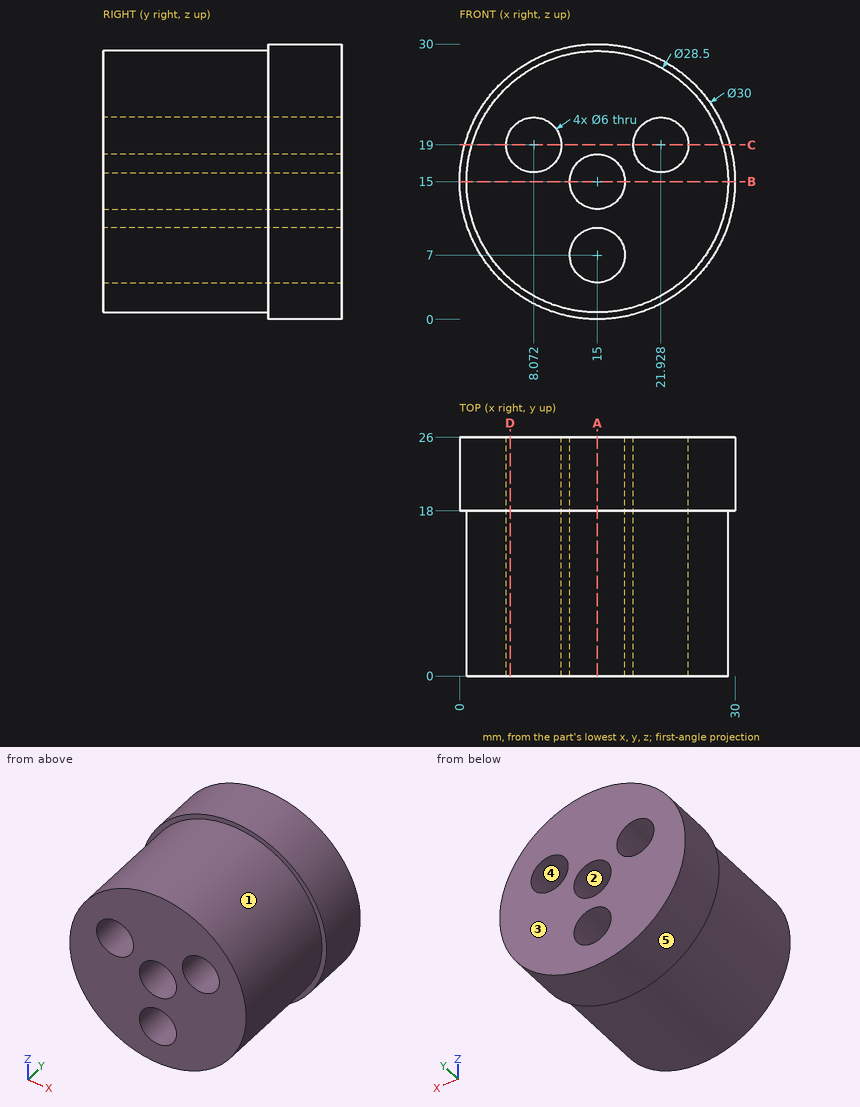
Geometry check sheet. Reference: drawing and pictorial views, mm from the part's lowest x, y, z. A direction names the side the tool comes from. Round coordinates to 2 decimals unless told otherwise and drop trailing zeros. Order: outer loops, then holes, each group sorted by start corner. A loop starts at its lowest first (then second) coordinate and runs counter-clockwise, first axis right, second up. Notation, with made-up numbers: (-5, -9.75) -> (31, -9.75) arc R17 cw to (31, 16.25) -> close; hole circle Ø3 at (15.25, -13.75). An arc over 180 degrees is marked (long way). One line per item, written item: value. Start each with the question number.
Q1. Thickness scan on line 1 (Z direction, x = 14, y = 21.25); line 2 (Z direction, x = 15.5, y = 2.25); line 3 (X direction, y = 8, z = 6). Record the ranges inside material, lowest first.
Q2. Cross-section at B-B (z = 15). Record the boundary of the cut face in (x, y), and give its area (3 significant figures).
Q3. Mould release check, pull along Z, two halves, no side actions. Record for the marked faces 3, 4 and 5: pulls with the +Z half, pulls with the -Z half, needs draft (parallel to the pull), parting line crosses it, or undercut.
Q4. Cross-section at D-D (x = 5.5). Record the boundary of the cut face in (y, z) (1 decimal), and give its area (3 significant figures).
Q5. Cross-section at C-C (z = 19). Record the boundary of the cut face in (x, y), and give its area (3 significant figures).
Q6. Cross-section at A-A (x = 15). Record the boundary of the cut face in (y, z), and give its area (3 significant figures).
Q7. Set-up check for the marked faces 1 and 2: record each of +Z, -Z, +X, -X, +Y, -Y from which the full face is reachable in a straight line by a thin tool's end or side.
Q8. Gauge pin test, flat ends, axial feed: pin 1 Ø1.5 at (y, z) = (13.5, 13) entering from -X (3 decimals); pin 2 Ø1.5 at (x, y) = (18, 8) entering from -Z; pin 3 Ø2 at (y, z) = (7.5, 24.5) entering from +X; pin 4 Ø5 at (x, z) = (21.93, 19) entering from -Y. Record the tip position at first contact, or that the pin passes through.
Completed:
1. line 1: z = 0.03 to 4.17, 9.83 to 12.17, 17.83 to 29.97
1. line 2: z = 0.76 to 4.04, 9.96 to 12.04, 17.96 to 29.24
1. line 3: x = 3.95 to 12.17, 17.83 to 26.05
2. outline: (0, 18) -> (0.75, 18) -> (0.75, 0) -> (12, 0) -> (12, 26) -> (0, 26) -> close; (18, 0) -> (29.25, 0) -> (29.25, 18) -> (30, 18) -> (30, 26) -> (18, 26) -> close
2. area: 597 mm²
3. face 3: needs draft
3. face 4: undercut
3. face 5: parting line crosses it
4. outline: (0, 4.4) -> (18, 4.4) -> (18, 3.4) -> (26, 3.4) -> (26, 17.5) -> (0, 17.5) -> close; (0, 20.5) -> (26, 20.5) -> (26, 26.6) -> (18, 26.6) -> (18, 25.6) -> (0, 25.6) -> close
4. area: 488 mm²
5. outline: (0.54, 18) -> (1.32, 18) -> (1.32, 0) -> (5.07, 0) -> (5.07, 26) -> (0.54, 26) -> close; (11.07, 0) -> (18.93, 0) -> (18.93, 26) -> (11.07, 26) -> close; (24.93, 0) -> (28.68, 0) -> (28.68, 18) -> (29.46, 18) -> (29.46, 26) -> (24.93, 26) -> close
5. area: 412 mm²
6. outline: (0, 0.75) -> (18, 0.75) -> (18, 0) -> (26, 0) -> (26, 4) -> (0, 4) -> close; (0, 10) -> (26, 10) -> (26, 12) -> (0, 12) -> close; (0, 18) -> (26, 18) -> (26, 30) -> (18, 30) -> (18, 29.25) -> (0, 29.25) -> close
6. area: 441 mm²
7. face 1: -Y
7. face 2: +Y, -Y
8. pin 1: stops at x = 0.805
8. pin 2: stops at z = 0.93
8. pin 3: stops at x = 26.44
8. pin 4: passes through
